The listing builds one solid part. Answer for the finished solid, in the listing's coordinates (mm). A direction names the side the tool comes from. Coordinates: 2 decimals unless noted, no trailing zeros. Order: outer loops, then holes, each group sorted by start corner. A loop starts at its lowest first (then second) coordinate and runs counter-clockwise, first axis right, second up.
from build123d import *

# Parameters (mm, degrees)
SKETCH_W        = 50
SKETCH_H        = 20
SKETCH_R        = 2.1
PAD_DEPTH       = 22
SKETCH001_R     = 11.2
POCKET_DEPTH    = 8
SKETCH002_R     = 5.1
SKETCH002_R_2   = 1.75
POCKET001_DEPTH = 20


with BuildPart() as part:
    # Sketch → Pad (new body)
    with BuildSketch(Plane.XY):
        with Locations((25, 10)):
            Rectangle(SKETCH_W, SKETCH_H)
        with Locations((10, 15)):
            Circle(SKETCH_R, mode=Mode.SUBTRACT)
        with Locations((10, 5)):
            Circle(SKETCH_R, mode=Mode.SUBTRACT)
        with Locations((40, 15)):
            Circle(SKETCH_R, mode=Mode.SUBTRACT)
        with Locations((40, 5)):
            Circle(SKETCH_R, mode=Mode.SUBTRACT)
    extrude(amount=PAD_DEPTH)

    # Sketch001 (on Face3 of Pad) → Pocket (cut)
    with BuildSketch(Plane.XZ):
        with Locations((25, 11)):
            Circle(SKETCH001_R)
    extrude(amount=-POCKET_DEPTH, mode=Mode.SUBTRACT)

    # Sketch002 (on Face1 of Pocket) → Pocket001 (cut)
    with BuildSketch(Plane(origin=(0, 20, 0), x_dir=(-1, 0, 0), z_dir=(0, 1, 0))):
        with Locations((-25, 11)):
            Circle(SKETCH002_R)
        with Locations((-25, 18.95)):
            Circle(SKETCH002_R_2)
        with Locations((-25, 3.05)):
            Circle(SKETCH002_R_2)
        with Locations((-32.95, 11)):
            Circle(SKETCH002_R_2)
        with Locations((-17.05, 11)):
            Circle(SKETCH002_R_2)
    extrude(amount=-POCKET001_DEPTH, mode=Mode.SUBTRACT)


solid = part.part
1) This flat-tipped pin is pushed along its axis until it touches: P1, Ø6.5, axis at x = 10, y = 5, coming from the +Z side. Where does it stop, or does it pass through?
2) Section C-C (y = 5) is taken. Give the vertices of the cut face in (x, z).
3) Determine the mould class of faces 3 (the face through (7.9, 5.09, 10.85)), 4 (the face through (7.9, 15.09, 10.85)), 5 (the face through (36.2, 3.9, 10.8)), 6 (the face through (19, 20, 11)) for opening direction Y: released by +Y, released by -Y, zero draft, split by the parting line, or undercut.
4) A tool of negligible diameter and unlimited length cuts with its end or side. For faces 1 (the face through (9, 0, 11)), 2 (the face through (13.8, 3.9, 11.2)), from which of +Z, -Z, +X, -X, +Y, -Y can it reach the whole face along a straight path? Write none if from no direction.
5) Section D-D (z = 11) is taken. Give the vertices of the cut face in (x, y), then the cut area to 3 significant figures.
6) Section A-A (y = 15) is taken. Give the vertices of the cut face in (x, z).
7) Consider L1, parallel to Z at x = 25, y = 15.5; L2, parallel to Y at x = 40, z = 7; L3, parallel to X at y = 14, z = 14. Determine where each line is inside the solid, lowest interval first.
8) Section B-B (x = 40) is taken. Give the vertices of the cut face in (y, z), then the cut area to 3 significant figures.
Filled sheet:
1. P1: stops at z = 22
2. outline: (0, 0) - (7.9, 0) - (7.9, 22) - (0, 22) - close; (12.1, 0) - (22.89, 0) arc R11.2 cw to (22.89, 22) - (12.1, 22) - close; (27.11, 0) - (37.9, 0) - (37.9, 22) - (27.11, 22) arc R11.2 cw to start; (42.1, 0) - (50, 0) - (50, 22) - (42.1, 22) - close
3. face 3: undercut
3. face 4: undercut
3. face 5: zero draft
3. face 6: released by +Y
4. face 1: +Z, -Z, +X, -X, -Y
4. face 2: -Y
5. outline: (0, 0) - (13.8, 0) - (13.8, 8) - (15.3, 8) - (15.3, 20) - (0, 20) - close; (18.8, 8) - (19.9, 8) - (19.9, 20) - (18.8, 20) - close; (30.1, 8) - (31.2, 8) - (31.2, 20) - (30.1, 20) - close; (34.7, 8) - (36.2, 8) - (36.2, 0) - (50, 0) - (50, 20) - (34.7, 20) - close; hole circle Ø4.2 at (10, 5); hole circle Ø4.2 at (10, 15); hole circle Ø4.2 at (40, 5); hole circle Ø4.2 at (40, 15)
5. area: 559 mm2
6. outline: (0, 0) - (7.9, 0) - (7.9, 22) - (0, 22) - close; (12.1, 0) - (37.9, 0) - (37.9, 22) - (12.1, 22) - close; (42.1, 0) - (50, 0) - (50, 22) - (42.1, 22) - close; hole circle Ø3.5 at (17.05, 11); hole circle Ø10.2 at (25, 11); hole circle Ø3.5 at (25, 3.05); hole circle Ø3.5 at (25, 18.95); hole circle Ø3.5 at (32.95, 11)
7. L1: z = 0 to 1.3, 4.8 to 5.9, 16.1 to 17.2, 20.7 to 22
7. L2: y = 0 to 2.9, 7.1 to 12.9, 17.1 to 20
7. L3: x = 0 to 8.15, 11.85 to 20.88, 29.12 to 38.15, 41.85 to 50
8. outline: (0, 0) - (2.9, 0) - (2.9, 22) - (0, 22) - close; (7.1, 0) - (12.9, 0) - (12.9, 22) - (7.1, 22) - close; (17.1, 0) - (20, 0) - (20, 22) - (17.1, 22) - close
8. area: 255 mm2
